Design review of the part built by this model. Coordinates are the model's own, in mm. Face numbers are marked on the shaded views. A direction names the side the tool comes from. Coordinates: 2 decimals unless noted, no trailing zeros. Order: outer loops, then holes, each group sorted by start corner. A loop starts at its lowest first (then second) coordinate and runs counter-clockwise, first axis right, second up. Notation, with made-up numbers: (88, 47.25) -> (137, 47.25) arc R35 ccw to (137, 81.25) -> close; hole circle Ø6 at (9, 76). An arc over 180 degrees is marked (long way). Use a Markdown table: item, result. Add a question column.
Q1. Add section C-C (x = 117). State the section outline as (y, z) points.
Q2. Insertion check: pin 1 (4 mm diameter, centred on y = -20.5, z = -118, fed in from +X); pin 2 (1 mm diameter, centred on x = 49.5, y = -16, fed in from -Z); pin 3 (3 mm diameter, centred on x = 104, y = -10, fed in from -Z). Each pin has a flat end and moves straight along its axis. Give the tip position at first contact, or say it passes through.
Q3. Wall thickness on probe 1 along Z at (x, y) = (28, -5); probe 2 along Z at (x, y) = (113, -4.75); probe 3 along X at (y, z) = (-12.75, -25.5): over which ranges is each line inside the solid? List them lowest first.
Q4. Add section A-A (y = -4.25). State the section outline as (x, z) points.
Q5. The part is to be moulded in two halves that separate along X. For the marked faces 1, 2 and 3, say which applies: pulls with the +X half, pulls with the -X half, needs draft (parallel to the pull), parting line crosses it, or undercut.
Q6. Machinability: for the marked faces 4 and 5, which of the approach directions +Z, -Z, +X, -X, +Y, -Y give a long, thin tool a straight path to every point of the face, cutting with its end or side? Answer none if there is none.
Q7. Add section B-B (z = -42). State the section outline as (x, y) points, then the cut area to 3 significant figures.
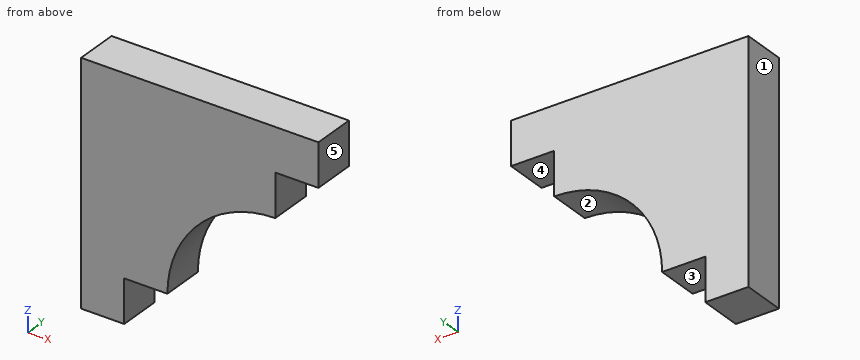
from build123d import *

# Parameters (mm, degrees)
F1_DEPTH = 25.4


with BuildPart() as f1:
    # F0 (on Front) → F1 (new body)
    with BuildSketch(Plane.XZ):
        with BuildLine():
            Line((139.7, 0), (0, 0))
            Line((0, 0), (0, -139.7))
            Line((0, -139.7), (25.4, -139.7))
            Line((25.4, -139.7), (25.4, -114.3))
            Line((25.4, -114.3), (50.8, -114.3))
            ThreePointArc((50.8, -114.3), (69.398719, -69.398719), (114.3, -50.8))
            Line((114.3, -50.8), (114.3, -25.4))
            Line((114.3, -25.4), (139.7, -25.4))
            Line((139.7, -25.4), (139.7, 0))
        make_face()
    extrude(amount=F1_DEPTH)


solid = f1.part
Established:
| question | item | result |
|---|---|---|
| 1 | outline | (-25.4, -25.4) -> (0, -25.4) -> (0, 0) -> (-25.4, 0) -> close |
| 2 | pin 1 | x = 25.4 |
| 2 | pin 2 | z = -114.3 |
| 2 | pin 3 | z = -51.91 |
| 3 | probe 1 | -114.3 to 0 |
| 3 | probe 2 | -50.81 to 0 |
| 3 | probe 3 | 0 to 114.3 |
| 4 | outline | (0, -139.7) -> (25.4, -139.7) -> (25.4, -114.3) -> (50.8, -114.3) arc R63.5 cw to (114.3, -50.8) -> (114.3, -25.4) -> (139.7, -25.4) -> (139.7, 0) -> (0, 0) -> close |
| 5 | face 1 | pulls with the -X half |
| 5 | face 2 | pulls with the +X half |
| 5 | face 3 | needs draft |
| 6 | face 4 | -Z, +X, +Y, -Y |
| 6 | face 5 | +Z, -Z, +X, +Y, -Y |
| 7 | outline | (0, -25.4) -> (114.3, -25.4) -> (114.3, 0) -> (0, 0) -> close |
| 7 | area | 2,900 mm^2 |
